```python
from build123d import *

# Parameters (mm, degrees)
F0_R     = 11.2
F1_DEPTH = 7


with BuildPart() as f1:
    # F0 (on Top) → F1 (new body)
    with BuildSketch(Plane.XY):
        with BuildLine():
            ThreePointArc((13.026173, 2.135137), (13.156472, 1.071101), (13.2, 0))
            ThreePointArc((13.2, 0), (13.156472, -1.071101), (13.026173, -2.135137))
            ThreePointArc((13.026173, -2.135137), (14.605448, -6.573318), (17.642623, -10.174308))
            ThreePointArc((17.642623, -10.174308), (20.336655, -10.92785), (22.492241, -12.710848))
            ThreePointArc((22.492241, -12.710848), (34.028768, -10.517447), (39.252346, 0))
            ThreePointArc((39.252346, 0), (33.297709, 11.033799), (20.806177, 12.112708))
            ThreePointArc((20.806177, 12.112708), (19.638047, 11.252162), (18.302422, 10.685442))
            ThreePointArc((18.302422, 10.685442), (14.818981, 6.93192), (13.026173, 2.135137))
        make_face()
        with Locations((26.052346, 0)):
            Circle(F0_R, mode=Mode.SUBTRACT)
        with BuildLine():
            ThreePointArc((2.335909, 12.991671), (9.405556, 9.261507), (13.026173, 2.135137))
            ThreePointArc((13.026173, 2.135137), (14.818981, 6.93192), (18.302422, 10.685442))
            ThreePointArc((18.302422, 10.685442), (12.328836, 12.090695), (10.464205, 17.9372))
            ThreePointArc((10.464205, 17.9372), (6.861144, 14.70661), (2.335909, 12.991671))
        make_face()
        with BuildLine():
            ThreePointArc((17.642623, -10.174308), (14.605448, -6.573318), (13.026173, -2.135137))
            ThreePointArc((13.026173, -2.135137), (9.552918, -9.109432), (2.751477, -12.910049))
            ThreePointArc((2.751477, -12.910049), (7.102679, -14.693916), (10.552385, -17.889956))
            ThreePointArc((10.552385, -17.889956), (12.254899, -12.338884), (17.642623, -10.174308))
        make_face()
        with BuildLine():
            ThreePointArc((-2.335909, 12.991671), (0, 13.2), (2.335909, 12.991671))
            ThreePointArc((2.335909, 12.991671), (6.861144, 14.70661), (10.464205, 17.9372))
            ThreePointArc((10.464205, 17.9372), (11.132538, 19.713613), (12.305166, 21.206013))
            ThreePointArc((12.305166, 21.206013), (12.974363, 23.553137), (13.2, 25.983343))
            ThreePointArc((13.2, 25.983343), (-1.911461, 39.044213), (-12.646411, 22.200715))
            ThreePointArc((-12.646411, 22.200715), (-11.342134, 20.393236), (-10.703132, 18.257868))
            ThreePointArc((-10.703132, 18.257868), (-7.03117, 14.811833), (-2.335909, 12.991671))
        make_face()
        with Locations((0, 25.983343)):
            Circle(F0_R, mode=Mode.SUBTRACT)
        with BuildLine():
            ThreePointArc((20.806177, 12.112708), (19.51523, 11.467611), (18.302422, 10.685442))
            ThreePointArc((18.302422, 10.685442), (19.638047, 11.252162), (20.806177, 12.112708))
        make_face()
        with BuildLine():
            ThreePointArc((10.552385, -17.889956), (7.102679, -14.693916), (2.751477, -12.910049))
            ThreePointArc((2.751477, -12.910049), (0, -13.2), (-2.751477, -12.910049))
            ThreePointArc((-2.751477, -12.910049), (-8.080001, -15.382016), (-11.808487, -19.920978))
            ThreePointArc((-11.808487, -19.920978), (-3.030509, -38.667512), (13.2, -25.820099))
            ThreePointArc((13.2, -25.820099), (13.039715, -23.769289), (12.562754, -21.768284))
            ThreePointArc((12.562754, -21.768284), (11.234444, -19.996615), (10.552385, -17.889956))
        make_face()
        with Locations((0, -25.820099)):
            Circle(F0_R, mode=Mode.SUBTRACT)
        with BuildLine():
            ThreePointArc((22.492241, -12.710848), (20.336655, -10.92785), (17.642623, -10.174308))
            ThreePointArc((17.642623, -10.174308), (19.934527, -11.696679), (22.492241, -12.710848))
        make_face()
        with BuildLine():
            ThreePointArc((-12.998967, 2.294961), (-9.348503, 9.319092), (-2.335909, 12.991671))
            ThreePointArc((-2.335909, 12.991671), (-7.03117, 14.811833), (-10.703132, 18.257868))
            ThreePointArc((-10.703132, 18.257868), (-12.70956, 12.601772), (-18.441334, 10.823021))
            ThreePointArc((-18.441334, 10.823021), (-14.870725, 7.10107), (-12.998967, 2.294961))
        make_face()
        with BuildLine():
            ThreePointArc((12.305166, 21.206013), (11.132538, 19.713613), (10.464205, 17.9372))
            ThreePointArc((10.464205, 17.9372), (11.501406, 19.50587), (12.305166, 21.206013))
        make_face()
        with BuildLine():
            ThreePointArc((-11.808487, -19.920978), (-8.080001, -15.382016), (-2.751477, -12.910049))
            ThreePointArc((-2.751477, -12.910049), (-9.496797, -9.167925), (-12.998967, -2.294961))
            ThreePointArc((-12.998967, -2.294961), (-15.519744, -8.027921), (-20.399145, -11.953809))
            ThreePointArc((-20.399145, -11.953809), (-13.49629, -13.12581), (-11.808487, -19.920978))
        make_face()
        with BuildLine():
            ThreePointArc((12.562754, -21.768284), (11.71912, -19.745379), (10.552385, -17.889956))
            ThreePointArc((10.552385, -17.889956), (11.234444, -19.996615), (12.562754, -21.768284))
        make_face()
        with BuildLine():
            ThreePointArc((-12.998967, -2.294961), (-13.2, 0), (-12.998967, 2.294961))
            ThreePointArc((-12.998967, 2.294961), (-14.870725, 7.10107), (-18.441334, 10.823021))
            ThreePointArc((-18.441334, 10.823021), (-20.327157, 11.431359), (-21.952488, 12.564807))
            ThreePointArc((-21.952488, 12.564807), (-39.178277, -0.720131), (-20.607655, -12.049269))
            ThreePointArc((-20.607655, -12.049269), (-20.503828, -12.000604), (-20.399145, -11.953809))
            ThreePointArc((-20.399145, -11.953809), (-15.519744, -8.027921), (-12.998967, -2.294961))
        make_face()
        with Locations((-25.997935, 0)):
            Circle(F0_R, mode=Mode.SUBTRACT)
        with BuildLine():
            ThreePointArc((-12.646411, 22.200715), (-11.840051, 20.147831), (-10.703132, 18.257868))
            ThreePointArc((-10.703132, 18.257868), (-11.342134, 20.393236), (-12.646411, 22.200715))
        make_face()
        with BuildLine():
            ThreePointArc((-21.952488, 12.564807), (-20.327157, 11.431359), (-18.441334, 10.823021))
            ThreePointArc((-18.441334, 10.823021), (-20.131903, 11.82496), (-21.952488, 12.564807))
        make_face()
        with BuildLine():
            ThreePointArc((-20.607655, -12.049269), (-20.503193, -12.001992), (-20.399145, -11.953809))
            ThreePointArc((-20.399145, -11.953809), (-20.503828, -12.000604), (-20.607655, -12.049269))
        make_face()
    extrude(amount=F1_DEPTH)


solid = f1.part
```
CAD build for the part. Positions are in the model's coordinates, mm. A direction names the side the tool comes from. Round coordinates to 2 decimals unless told otherwise and drop trailing zeros. Write each loop counter-clockwise with the first axis right and the second up, starting at its lowest first coordinate (ties: lowest second). Pieces come first, ordered by that corner, then holes.
Item 1: Tool access for faces 4 (the cylindrical face through (11.73, -19.77, 3.45)), 5 (the cylindrical face through (9.63, -9.03, 3.45)), 6 (the cylindrical face through (19.9, -11.68, 3.45)), 7 (the cylindrical face through (-11.854, 20.176, 3.451)): list every direction of +Z, -Z, +X, -X, +Y, -Y with a clear straight run to the whole face (end or side of a thin tool).
Filled in:
face 4: +Z, -Z, +X
face 5: +Z, -Z
face 6: +Z, -Z, -Y
face 7: +Z, -Z, -X
Item 2: Band-saw the part on B-B on y = -34. Write the cut outline in (x, z).
Filled in:
outline: (-10.36, 0) - (-7.65, 0) - (-7.65, 7) - (-10.36, 7) - close; (7.65, 0) - (10.36, 0) - (10.36, 7) - (7.65, 7) - close
Item 3: Drill centre lines: L1, parallel to X at y = 26.5, z = 6.75; L2, parallel to Y at x = 0.5, z = 2; L3, parallel to X at y = -5, z = 3. Where is each one in solid material? Low to high.
Filled in:
L1: x = -13.19 to -11.19, 11.19 to 13.19
L2: y = -39.01 to -37.01, -14.63 to -13.19, 13.19 to 14.79, 37.17 to 39.17
L3: x = -38.21 to -36.02, -15.98 to -12.22, 12.22 to 16.03, 36.07 to 38.27
Item 4: Mould opens along X. For faces 1 (the flat face through (-12, 6, 7)), 2 (the cylindrical face through (-1.458, -14.715, 3.451)), 3 (the cylindrical face through (13.044, -23.798, 3.451)) say: released by +X, released by -X, zero draft, split by the parting line, or undercut.
Filled in:
face 1: zero draft
face 2: undercut
face 3: released by +X
Item 5: Drop flat-ended pins along their axis: pin 1 Ø1 at (y, z) = (-17.5, 1) entering from -X; pin 2 Ø1.5 at (x, z) = (17, 2.5) entering from +Y; pin 3 Ø1.5 at (y, z) = (29.5, 1) entering from -X. Give the stop position or say it passes through.
Filled in:
pin 1: stops at x = -11.5
pin 2: stops at y = 10.55
pin 3: stops at x = -12.91
Item 6: Band-saw the part on D-D on x = 25. Write the cut outline in (y, z).
Filled in:
outline: (-13.16, 0) - (-11.15, 0) - (-11.15, 7) - (-13.16, 7) - close; (11.15, 0) - (13.16, 0) - (13.16, 7) - (11.15, 7) - close
Item 7: Band-saw the part on C-C on z = 3. Give the number of separate pieces and of enclosed holes in the cut face, then the cut area to 3 significant figures.
Filled in:
separate pieces: 1
enclosed holes: 5
area: 878 mm2
Item 8: Band-saw the part on A-A on x = 0. Write the cut outline in (y, z), then the cut area to 3 significant figures.
Filled in:
outline: (-39.02, 0) - (-37.02, 0) - (-37.02, 7) - (-39.02, 7) - close; (-14.62, 0) - (-13.2, 0) - (-13.2, 7) - (-14.62, 7) - close; (13.2, 0) - (14.78, 0) - (14.78, 7) - (13.2, 7) - close; (37.18, 0) - (39.18, 0) - (39.18, 7) - (37.18, 7) - close
area: 49.0 mm2
